The listing builds one solid part. Answer for the finished solid, in the listing's coordinates (mm). Face numbers are marked on the shaded views. A direction names the side the tool comes from. Coordinates: 2 decimals unless noted, no trailing zeros. Order: outer loops, then holes, each group sorted by start corner. A loop starts at its lowest first (then second) coordinate and runs counter-clockwise, first axis right, second up.
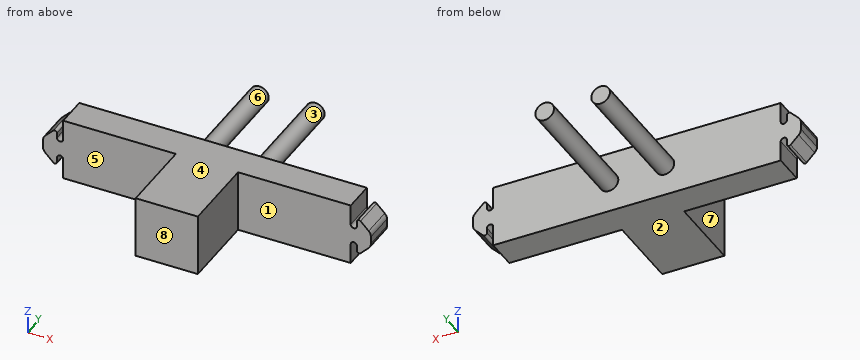
```python
from build123d import *

# Parameters (mm, degrees)
SKETCH1_W           = 117.475
SKETCH1_H           = 25.4
BOSS_EXTRUDE1_DEPTH = 12.7
SKETCH3_R           = 3.81
BOSS_EXTRUDE2_DEPTH = 50.8
BOSS_EXTRUDE7_DEPTH = 12.7
SKETCH12_W          = 25.4
SKETCH12_H          = 25.4
BOSS_EXTRUDE8_DEPTH = 31.75


with BuildPart() as part:
    # Sketch1 → Boss-Extrude1 (new body)
    with BuildSketch(Plane(origin=(0, 0, 0), x_dir=(1, 0, 0), z_dir=(0, 1, 0))):
        with Locations((-58.7375, -12.7)):
            Rectangle(SKETCH1_W, SKETCH1_H)
    extrude(amount=BOSS_EXTRUDE1_DEPTH)

    # Sketch3 → Boss-Extrude2 (add)
    with BuildSketch(Plane(origin=(0, 12.7, 0), x_dir=(1, 0, 0), z_dir=(0, 1, 0))):
        with Locations(Location((-47.3075, -12.7, 0), (0, 0, 270))):
            Circle(SKETCH3_R)
        with Locations(Location((-70.1675, -12.7, 0), (0, 0, 90))):
            Circle(SKETCH3_R)
    extrude(amount=BOSS_EXTRUDE2_DEPTH)

    # Sketch10 → Boss-Extrude7 (add)
    with BuildSketch(Plane(origin=(0, 12.7, 0), x_dir=(1, 0, 0), z_dir=(0, 1, 0))):
        with BuildLine():
            Line((0, -12.7), (0, -8.3566))
            ThreePointArc((0, -8.3566), (1.27, -9.6266), (2.54, -8.3566))
            Line((2.54, -8.3566), (2.54, -6.223))
            ThreePointArc((2.54, -6.223), (3.073114588, -5.425137636), (4.014257416, -5.612342584))
            Line((4.014257416, -5.612342584), (7.336952181, -8.935037349))
            ThreePointArc((7.336952181, -8.935037349), (8.017998618, -9.969860776), (8.2511937, -11.186538149))
            Line((8.2511937, -11.186538149), (8.2511937, -12.7))
            Line((8.2511937, -12.7), (0, -12.7))
        make_face()
        with BuildLine():
            Line((-117.475, -12.7), (-117.475, -8.3566))
            ThreePointArc((-117.475, -8.3566), (-118.745, -9.6266), (-120.015, -8.3566))
            Line((-120.015, -8.3566), (-120.015, -6.223))
            ThreePointArc((-120.015, -6.223), (-120.548114588, -5.425137636), (-121.489257416, -5.612342584))
            Line((-121.489257416, -5.612342584), (-124.811952181, -8.935037349))
            ThreePointArc((-124.811952181, -8.935037349), (-125.492998618, -9.969860776), (-125.7261937, -11.186538149))
            Line((-125.7261937, -11.186538149), (-125.7261937, -12.7))
            Line((-125.7261937, -12.7), (-117.475, -12.7))
        make_face()
    boss_extrude7 = extrude(amount=-BOSS_EXTRUDE7_DEPTH)

    # Mirror1: Boss-Extrude7 across plane
    add(boss_extrude7.mirror(Plane(origin=(8.2511937, 0, 12.7), x_dir=(1, 0, 0), z_dir=(0, 0, 1))))

    # Sketch12 → Boss-Extrude8 (add)
    with BuildSketch(Plane(origin=(0, 0, 0), x_dir=(-1, 0, 0), z_dir=(0, -1, 0))):
        with Locations((58.7375, -12.7)):
            Rectangle(SKETCH12_W, SKETCH12_H)
    extrude(amount=BOSS_EXTRUDE8_DEPTH)


solid = part.part
```
(1) Find section C-C (x = -9). Write down the section's boundary in (y, z), and give its area (3 significant figures).
(2) Find section A-A (y = 2.5). Write down the section's boundary in (x, z) (3 decimals), and give its area (3 significant figures).
(3) For the marked faces 1, 2, 3, 4 and 5, determine the directions among +Z, -Z, +X, -X, +Y, -Y from which every point of the face is accessible in a straight line to the end or side of a thin tool.
(4) Consider line 1 (X direction, y = 58.5, z = 12.75); line 2 (Y direction, x = -8, z = 7.5); line 3 (X direction, y = -26.5, z = 8.75). Determine where each line is inside the solid, lowest interval first.
(5) Find section B-B (z = 12.7). Write down the section's boundary in (x, y), and give its area (3 significant figures).
(6) The mould has two halves that part along X. Classify the marked faces 6, 7 and 8: released by +X, released by -X, zero draft, split by the parting line, or undercut.
(7) Find section D-D (y = 53.5). Write down the section's boundary in (x, z), and give its area (3 significant figures).
(8) Each of these flat-tipped pins is pushed along its axis until it touches: pin 1 Ø6.5 at (y, z) = (6, 4) entering from -X; pin 2 Ø12.5 at (y, z) = (-19, 12) entering from -X; pin 3 Ø4 at (y, z) = (30.5, 10.5) entering from +X; pin 4 Ø4 at (x, y) = (-108.5, 2.5) entering from -Z. Where does it stop, or does it pass through?
Findings below:
1. outline: (0, 0) - (12.7, 0) - (12.7, 25.4) - (0, 25.4) - close
1. area: 323 mm2
2. outline: (-125.726, 11.187) arc R3.175 ccw to (-124.812, 8.935) - (-121.489, 5.612) arc R0.864 ccw to (-120.015, 6.223) - (-120.015, 8.357) arc R1.27 cw to (-117.475, 8.357) - (-117.475, 0) - (0, 0) - (0, 8.357) arc R1.27 cw to (2.54, 8.357) - (2.54, 6.223) arc R0.864 ccw to (4.014, 5.612) - (7.337, 8.935) arc R3.175 ccw to (8.251, 11.187) - (8.251, 14.213) arc R3.175 ccw to (7.337, 16.465) - (4.014, 19.788) arc R0.864 ccw to (2.54, 19.177) - (2.54, 17.043) arc R1.27 cw to (0, 17.043) - (0, 25.4) - (-117.475, 25.4) - (-117.475, 17.043) arc R1.27 cw to (-120.015, 17.043) - (-120.015, 19.177) arc R0.864 ccw to (-121.489, 19.788) - (-124.812, 16.465) arc R3.175 ccw to (-125.726, 14.213) - close
2. area: 3,140 mm2
3. face 1: +Z, -Z, +X, -Y
3. face 2: -Z, +X, -X, +Y, -Y
3. face 3: +Y
3. face 4: +Z, +X, -X, +Y, -Y
3. face 5: +Z, -Z, -X, -Y
4. line 1: x = -73.98 to -66.36, -51.12 to -43.5
4. line 2: y = 0 to 12.7
4. line 3: x = -71.44 to -46.04
5. outline: (-125.73, 0) - (-71.44, 0) - (-71.44, -31.75) - (-46.04, -31.75) - (-46.04, 0) - (8.25, 0) - (8.25, 12.7) - (-43.5, 12.7) - (-43.5, 63.5) - (-51.12, 63.5) - (-51.12, 12.7) - (-66.36, 12.7) - (-66.36, 63.5) - (-73.98, 63.5) - (-73.98, 12.7) - (-125.73, 12.7) - close
5. area: 3,280 mm2
6. face 6: undercut
6. face 7: released by -X
6. face 8: zero draft
7. outline: circle Ø7.62 at (-70.17, 12.7); circle Ø7.62 at (-47.31, 12.7)
7. area: 91.2 mm2
8. pin 1: stops at x = -123.13
8. pin 2: stops at x = -71.44
8. pin 3: stops at x = -43.5
8. pin 4: stops at z = 0
